Work out the finished part from the listing and answer in its coordinate system (mm). Give positions to 0.01 mm unless a question says otherwise; leave off trailing zeros. Order: outer loops, then holes, each group sorted by start corner. A loop starts at its lowest first (then second) coordinate and runs counter-clockwise, first axis right, second up. Notation, with made-up numbers: (-31, 20.5) -> (6, 20.5) arc R13 ccw to (6, 40.5) -> close; hole circle Ø8 at (88, 2.5). An arc over 180 degrees is marked (long way). Answer as CSV lines item,"result". Start each with the question number.
1. A cutting plane is placed at B-B (x = -61.5). Give the vertices of the cut face in (y, z), then the cut area to 3 significant figures.
2. Find the intervals of material crossed by L1, parallel to Y at x = -38, z = 1.45; L2, parallel to Y at x = -33.5, z = 4.7; L3, parallel to Y at x = -75, z = 2.25, in increasing order.
3. Flat-ended cylindrical pins translate along their axes: pin 1 (2.5 mm diameter, centred on x = -37.87, y = 65.6, fed in from -Z) (3 decimals); pin 2 (2 mm diameter, centred on y = 8, z = 2, fed in from +X). Find the tip coordinate at first contact, or state that the pin passes through.
4. A cutting plane is placed at A-A (z = 2.1). Give the vertices of the cut face in (x, y) (3 decimals).
5. A cutting plane is placed at C-C (y = -59). Give the vertices of the cut face in (x, z), then the cut area to 3 significant figures.
from build123d import *

# Parameters (mm, degrees)
F1_DEPTH = 5.08
F3_DEPTH = 25.4
F5_DEPTH = 25.4
F7_DEPTH = 25.4


with BuildPart() as f1:
    # F0 (on Top) → F1 (new body)
    with BuildSketch(Plane.XY):
        Polygon((43.9928, 76.197765), (-43.9928, 76.197765), (-87.9856, 0), (-43.9928, -76.197765), (43.9928, -76.197765), (87.9856, 0), align=None)
    extrude(amount=F1_DEPTH)

    # F2 (on face) → F3 (cut)
    with BuildSketch(Plane.XY.offset(5.08)):
        with BuildLine():
            ThreePointArc((-38.6969, 67.024997), (-38.6969, 64.165381), (-36.2204, 65.595189))
            ThreePointArc((-36.2204, 65.595189), (-37.0459, 67.024997), (-38.6969, 67.024997))
        make_face()
        with BuildLine():
            ThreePointArc((38.6969, 67.024997), (36.441592, 64.769689), (39.5224, 65.595189))
            ThreePointArc((39.5224, 65.595189), (39.301208, 66.420689), (38.6969, 67.024997))
        make_face()
        with BuildLine():
            ThreePointArc((38.6969, -67.024997), (39.301208, -66.420689), (39.5224, -65.595189))
            ThreePointArc((39.5224, -65.595189), (36.441592, -64.769689), (38.6969, -67.024997))
        make_face()
        with BuildLine():
            ThreePointArc((-38.6969, -67.024997), (-37.0459, -67.024997), (-36.2204, -65.595189))
            ThreePointArc((-36.2204, -65.595189), (-38.6969, -64.165381), (-38.6969, -67.024997))
        make_face()
    extrude(amount=-F3_DEPTH, mode=Mode.SUBTRACT)

    # F4 (on face) → F5 (cut)
    with BuildSketch(Plane.XY.offset(5.08)):
        with BuildLine():
            ThreePointArc((32.6898, -46.098765), (33.857233, -45.615198), (34.3408, -44.447765))
            ThreePointArc((34.3408, -44.447765), (31.522367, -43.280331), (32.6898, -46.098765))
        make_face()
    extrude(amount=-F5_DEPTH, mode=Mode.SUBTRACT)

    # F6 (on face) → F7 (cut)
    with BuildSketch(Plane.XY.offset(5.08)):
        with BuildLine():
            ThreePointArc((-31.0388, -52.385265), (-33.857233, -51.217831), (-32.6898, -54.036265))
            ThreePointArc((-32.6898, -54.036265), (-31.522367, -53.552698), (-31.0388, -52.385265))
        make_face()
    extrude(amount=-F7_DEPTH, mode=Mode.SUBTRACT)


solid = f1.part
Answer sheet:
1,outline,"(-45.87, 0) -> (45.87, 0) -> (45.87, 5.08) -> (-45.87, 5.08) -> close"
1,area,"466 mm^2"
2,L1,"y = -76.2 to -67.24, -63.95 to 63.95, 67.24 to 76.2"
2,L2,"y = -76.2 to -53.82, -50.95 to 76.2"
2,L3,"y = -22.49 to 22.49"
3,pin 1,"passes through"
3,pin 2,"stops at x = 83.94"
4,outline,"(-87.986, 0) -> (-43.993, -76.198) -> (43.993, -76.198) -> (87.986, 0) -> (43.993, 76.198) -> (-43.993, 76.198) -> close; hole circle Ø3.302 at (-37.871, -65.595); hole circle Ø3.302 at (-37.871, 65.595); hole circle Ø3.302 at (-32.69, -52.385); hole circle Ø3.302 at (32.69, -44.448); hole circle Ø3.302 at (37.871, -65.595); hole circle Ø3.302 at (37.871, 65.595)"
5,outline,"(-53.92, 0) -> (53.92, 0) -> (53.92, 5.08) -> (-53.92, 5.08) -> close"
5,area,"548 mm^2"
